from build123d import *

# Parameters (mm, degrees)
BOSS_EXTRUDE1_DEPTH = 3.175


with BuildPart() as part:
    # Sketch1 → Boss-Extrude1 (new body)
    with BuildSketch(Plane.XY):
        with BuildLine():
            Line((0, 0), (100, 0))
            ThreePointArc((100, 0), (122, 22), (100, 44))
            Line((100, 44), (0, 44))
            Line((0, 44), (0, 0))
        make_face()
        with BuildLine():
            Line((40, 2), (40, 42))
            Line((40, 42), (100, 42))
            ThreePointArc((100, 42), (120, 22), (100, 2))
            Line((100, 2), (40, 2))
        make_face(mode=Mode.SUBTRACT)
    extrude(amount=BOSS_EXTRUDE1_DEPTH)


solid = part.part
Read the model definition and answer for the solid it produces. Units are mm, in the model's axes. A direction names the side the tool comes from. Coordinates: 2 decimals unless noted, no trailing zeros. Write each loop counter-clockwise with the first axis right and the second up, starting at its lowest first coordinate (ties: lowest second). Pieces come first, ordered by that corner, then holes. Notation, with made-up numbers: M 53,-29 L 103,-29 A20 ccw 103,-18 Z; hole C 20,19 d7. An arc over 180 degrees is marked long. Use a Markdown table: item, result.
Q1. The part is cut by section B-B, the plane x = 85. Write down the section's boundary in (y, z) (3 decimals).
Answer block:
| item | result |
|---|---|
| outline | M 0,0 L 2,0 L 2,3.175 L 0,3.175 Z; M 42,0 L 44,0 L 44,3.175 L 42,3.175 Z |
Q2. The part is cut by section C-C, the plane z = 1. Write down the section's boundary in (x, y).
Answer block:
| item | result |
|---|---|
| outline | M 0,0 L 100,0 A22 ccw 100,44 L 0,44 Z; hole M 40,2 L 100,2 A20 ccw 100,42 L 40,42 Z |
Q3. This flat-tipped pin is pushed along its axis until it touches: pin 1 Ø1.5 at (x, z) = (101, 2.5) entering from +Y. Where does it stop, or does it pass through?
Answer block:
| item | result |
|---|---|
| pin 1 | stops at y = 44 |
Q4. Which of the six approach directions +Z, -Z, +X, -X, +Y, -Y give full straight-line access (tool end or side, diameter ignored) to faces 1 (the face through (29, 24, 0)), 2 (the face through (40, 22, 2))?
Answer block:
| item | result |
|---|---|
| face 1 | -Z, +X, -X, +Y, -Y |
| face 2 | +Z, -Z |
Q5. Determine the mould class of faces 3 (the face through (120, 22, 2)), 4 (the face through (122, 22, 2)), 5 (the face through (51, 44, 2)) for opening direction X: released by +X, released by -X, zero draft, split by the parting line, or undercut.
Answer block:
| item | result |
|---|---|
| face 3 | undercut |
| face 4 | released by +X |
| face 5 | zero draft |
Q6. Straight lines are drawn through the part: L1, parallel to Y at x = 61.5, z = 0.7; L2, parallel to X at y = 21, z = 3; L3, parallel to X at y = 12.5, z = 1.25. For each, find the intervals that lie inside material, in ascending order. Write a range as [from, to].
Answer block:
| item | result |
|---|---|
| L1 | y = [0, 2], [42, 44] |
| L2 | x = [0, 40], [119.97, 121.98] |
| L3 | x = [0, 40], [117.6, 119.84] |
Q7. The part is cut by section A-A, the plane y = 22. Write down the section's boundary in (x, z) (3 decimals), then the cut area to 3 significant figures.
Answer block:
| item | result |
|---|---|
| outline | M 0,0 L 40,0 L 40,3.175 L 0,3.175 Z; M 120,0 L 122,0 L 122,3.175 L 120,3.175 Z |
| area | 133 mm2 |
